Read the model definition and answer for the solid it produces. Units are mm, in the model's axes. A direction names the side the tool comes from. Give positions to 0.01 mm unless a question says otherwise; leave off trailing zeros. Write each loop counter-clockwise with the first axis right and the second up, starting at its lowest first coordinate (ties: lowest second). Pieces come first, ordered by that corner, then holes. Notation, with made-up numbers: (-34.75, -30) -> (-19.75, -30) arc R34 ccw to (-19.75, 0) -> close; hole circle Ø4 at (54, 35). An arc over 180 degrees is marked (long way). Answer as CSV lines item,"result". Start each with the question number.
1. For a pull along Y with two mould halves and no side action, classify faces 1 (the flat face through (-18.783, 7.443, 4.569)), 2 (the flat face through (-19, 10.16, -4)), 3 (the flat face through (0, 14, 0)) as pulls with the +Y half, pulls with the -Y half, needs draft (parallel to the pull), parting line crosses it, or undercut.
2. The part is cut by section D-D, the plane z = -11. Determine the outline of the cut face in (x, y), and give its area (3 significant figures).
3. The part is cut by section C-C, the plane x = -13. Determine the outline of the cut face in (y, z), and give its area (3 significant figures).
4. The part is cut by section B-B, the plane z = -3.25. Determine the outline of the cut face in (x, y).
5. A tool of negligible diameter and unlimited length cuts with its end or side. For faces 4 (the flat face through (-19, 10.16, 4)), 5 (the flat face through (-18.783, 7.378, -4.513)), 6 (the flat face through (-19, 12.7, -8)), 7 (the cylindrical face through (-33.336, 17.189, -0.219)), from which of +Z, -Z, +X, -X, +Y, -Y can it reach the whole face along a straight path? Write none if from no direction.
6. Given pin 1 (3 mm diameter, centred on x = -20.5, z = -5, fed in from +Y); pin 2 (3 mm diameter, centred on y = 17.5, z = 7.5, fed in from +X); pin 3 (3 mm diameter, centred on x = -13.5, z = -9, fed in from -Y); pin 4 (5 mm diameter, centred on x = -33.5, z = 7.5, fed in from -Y), each flat-ended and moving along its own axis, determine where each tip first touches the part or whether it passes through.
7. Find the intervals of material crossed by line 1 (Y direction, x = -14, z = 10.75); line 2 (Y direction, x = -29.5, z = -1.25); line 3 (Z direction, x = -30, y = 18), in increasing order.
from build123d import *

# Parameters (mm, degrees)
SKETCH10_W          = 5.08
SKETCH10_H          = 2.54
BOSS_EXTRUDE3_DEPTH = 38.1
SKETCH11_W          = 38.1
SKETCH11_H          = 25.4
BOSS_EXTRUDE4_DEPTH = 7.62
SKETCH12_R          = 14.2875
CUT_EXTRUDE1_DEPTH  = 6.35


with BuildPart() as part:
    # Sketch10 → Boss-Extrude3 (new body)
    with BuildSketch(Plane(origin=(0, 0, 0), x_dir=(0, 0, -1), z_dir=(1, 0, 0))):
        with BuildLine():
            Line((6.35, 10.16), (-6.35, 10.16))
            ThreePointArc((-6.35, 10.16), (-6.580814495, 10.012022021), (-6.542688341, 9.740509205))
            Line((-6.542688341, 9.740509205), (-2.54, 5.08))
            Line((-2.54, 5.08), (2.54, 5.08))
            Line((2.54, 5.08), (6.542688341, 9.740509205))
            ThreePointArc((6.542688341, 9.740509205), (6.580814495, 10.012022021), (6.35, 10.16))
        make_face()
        with Locations((0, 11.43)):
            Rectangle(SKETCH10_W, SKETCH10_H)
    extrude(amount=-BOSS_EXTRUDE3_DEPTH)

    # Sketch11 → Boss-Extrude4 (add)
    with BuildSketch(Plane(origin=(0, 12.7, 0), x_dir=(1, 0, 0), z_dir=(0, 1, 0))):
        with Locations((-19.05, 0)):
            Rectangle(SKETCH11_W, SKETCH11_H)
    extrude(amount=BOSS_EXTRUDE4_DEPTH)

    # Sketch12 → Cut-Extrude1 (cut)
    with BuildSketch(Plane(origin=(0, 20.32, 0), x_dir=(1, 0, 0), z_dir=(0, 1, 0))):
        with Locations((-19.05, 0)):
            Circle(SKETCH12_R)
    extrude(amount=-CUT_EXTRUDE1_DEPTH, mode=Mode.SUBTRACT)


solid = part.part
Results found:
1,face 1,"pulls with the -Y half"
1,face 2,"undercut"
1,face 3,"needs draft"
2,outline,"(-38.1, 12.7) -> (0, 12.7) -> (0, 20.32) -> (-9.93, 20.32) -> (-9.93, 13.97) -> (-28.17, 13.97) -> (-28.17, 20.32) -> (-38.1, 20.32) -> close"
2,area,"175 mm²"
3,outline,"(5.08, -2.54) -> (9.74, -6.54) arc R0.25 ccw to (10.16, -6.35) -> (10.16, -2.54) -> (12.7, -2.54) -> (12.7, -12.7) -> (13.97, -12.7) -> (13.97, 12.7) -> (12.7, 12.7) -> (12.7, 2.54) -> (10.16, 2.54) -> (10.16, 6.35) arc R0.25 ccw to (9.74, 6.54) -> (5.08, 2.54) -> close"
3,area,"93.0 mm²"
4,outline,"(-38.1, 5.91) -> (0, 5.91) -> (0, 10.16) -> (-38.1, 10.16) -> close; (-38.1, 12.7) -> (0, 12.7) -> (0, 20.32) -> (-5.14, 20.32) -> (-5.14, 13.97) -> (-32.96, 13.97) -> (-32.96, 20.32) -> (-38.1, 20.32) -> close"
5,face 4,"+Z, +X, -X"
5,face 5,"-Z, +X, -X, -Y"
5,face 6,"-Z, +X, -X"
5,face 7,"+Y"
6,pin 1,"stops at y = 13.97"
6,pin 2,"stops at x = 0"
6,pin 3,"stops at y = 12.7"
6,pin 4,"stops at y = 7.94"
7,line 1,"y = 12.7 to 13.97"
7,line 2,"y = 5.08 to 13.97"
7,line 3,"z = -12.7 to -9.18, 9.18 to 12.7"
